Source: three-view drawing plus pictorial views. Frame: mm from the lowest corner of the part. Round coordinates to 2 decimals unless told otherwise and drop trailing zeros. Loops run counter-clockwise (first coordinate to the right, second up) from the corner with the lowest first, then second, coordinate; pieces in that order, holes last. Notation, with made-up numbers: (26.5, 75) -> (77.5, 75) arc R27 ccw to (77.5, 95) -> close; hole circle Ø2 at (-39.5, -19.5). An arc over 180 degrees is marked (long way). Answer in a Markdown table with one row per item. Add a question column.
Q1. Section B-B, the plane z = 1.7. Give the number of separate pieces and of enclosed holes in the cut face, and give its area (3 significant figures).
Q2. Ray query, L1, parallel to X at y = 77, z = 1.1; L2, parallel to Y at x = 68, z = 1.6. Return the intervals inside material, ascending. Write a range as from..to.
Q3. Pin query (flat end, axial travel): pin 1 (2.5 mm diameter, centred on x = 77, y = 58, fed in from +Z). Return the tip coordinate at first contact, or that it passes through.
Q4. Section D-D, the plane x = 77. Output: boundary loops of the cut face in (y, z).
Q5. Section A-A, the plane x = 12. Output: boundary loops of the cut face in (y, z).
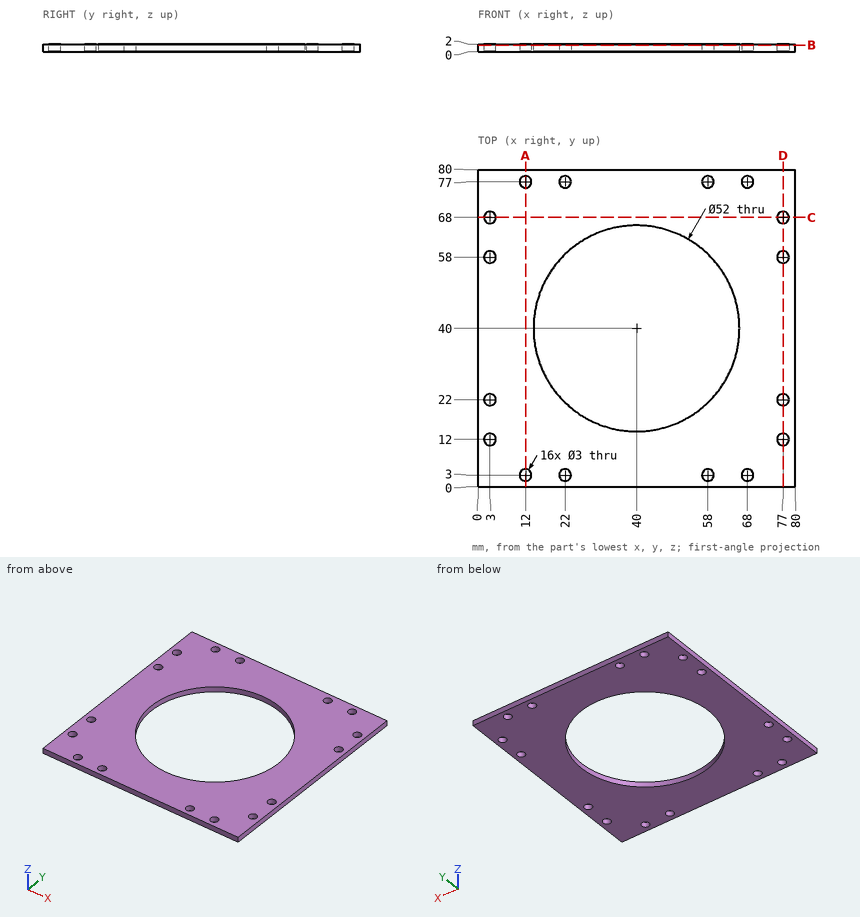
Answer block:
| question | item | result |
|---|---|---|
| 1 | separate pieces | 1 |
| 1 | enclosed holes | 17 |
| 1 | area | 4,160 mm^2 |
| 2 | L1 | 0..10.5, 13.5..20.5, 23.5..56.5, 59.5..66.5, 69.5..80 |
| 2 | L2 | 0..1.5, 4.5..75.5, 78.5..80 |
| 3 | pin 1 | through |
| 4 | outline | (0, 0) -> (10.5, 0) -> (10.5, 2) -> (0, 2) -> close; (13.5, 0) -> (20.5, 0) -> (20.5, 2) -> (13.5, 2) -> close; (23.5, 0) -> (56.5, 0) -> (56.5, 2) -> (23.5, 2) -> close; (59.5, 0) -> (66.5, 0) -> (66.5, 2) -> (59.5, 2) -> close; (69.5, 0) -> (80, 0) -> (80, 2) -> (69.5, 2) -> close |
| 5 | outline | (0, 0) -> (1.5, 0) -> (1.5, 2) -> (0, 2) -> close; (4.5, 0) -> (75.5, 0) -> (75.5, 2) -> (4.5, 2) -> close; (78.5, 0) -> (80, 0) -> (80, 2) -> (78.5, 2) -> close |
